Work out the finished part from the listing and answer in its coordinate system (mm). Round coordinates to 2 decimals unless told otherwise and drop trailing zeros. Order: outer loops, then holes, each group sorted by start corner. A loop starts at its lowest first (then second) coordinate and runs counter-clockwise, first axis right, second up. Notation, with made-up numbers: (48.5, -19.5) - (52.5, -19.5) arc R17 cw to (52.5, -1.5) - close; hole circle Ø4 at (88.5, 79). An arc over 180 degrees is marked (long way). Answer in a Markdown table with one row per item.
Autodesk Inventor part; units mm, degrees
ref_plane "YZ Plane" through (0, 0, 0) normal (1, 0, 0) x (0, 1, 0)
ref_plane "XZ Plane" through (0, 0, 0) normal (0, 1, 0) x (-1, 0, 0)
ref_plane "XY Plane" through (0, 0, 0) normal (0, 0, 1) x (1, 0, 0)
sketch "Sketch1" plane through (0, 0, 0) normal (0, 1, 0) x (-1, 0, 0)
  line L0 (0, 0) -> (40, 0)
  line L1 (40, 0) -> (40, -40)
  line L2 (40, -40) -> (0, -40)
  line L3 (0, -15.101) -> (0, 0)
  line L4 (0, -24.899) -> (0, -40)
  arc A0 (0, -24.899) -> (0, -15.101) centre (5.8365, -20) ccw
  dimension "d0" = 40
  dimension "d1" = 40
  dimension "d7" = 7.62
extrude "Extrusion1" add sketch "Sketch1" along normal blind 40
properties part number "railblock"
1) Find section C-C, the plane x = -3. Give the vertices of the cut face in (y, z).
Filled in:
| item | result |
|---|---|
| outline | (0, -40) - (40, -40) - (40, -27.07) - (0, -27.07) - close; (0, -12.93) - (40, -12.93) - (40, 0) - (0, 0) - close |
2) Find section A-A, the plane z = -27. Give the vertices of the cut face in (x, y), then the cut area to 3 significant figures.
Filled in:
| item | result |
|---|---|
| outline | (-40, 0) - (-8.85, 0) - (-8.85, 40) - (-40, 40) - close; (-2.83, 0) - (0, 0) - (0, 40) - (-2.83, 40) - close |
| area | 1,360 mm^2 |
3) Find section B-B, the plane y = 18.5. Give the vertices of the cut face in (x, z).
Filled in:
| item | result |
|---|---|
| outline | (-40, -40) - (0, -40) - (0, -24.9) arc R7.62 cw (long way) to (0, -15.1) - (0, 0) - (-40, 0) - close |
4) Find section D-D, the plane z = -20. Give the vertices of the cut face in (x, y).
Filled in:
| item | result |
|---|---|
| outline | (-40, 0) - (-13.46, 0) - (-13.46, 40) - (-40, 40) - close |
5) Find the intervals of material crossed by probe 1 along X at (y, z) = (31, -20); probe 2 along Z at (x, y) = (-3.5, 37); probe 3 along X at (y, z) = (13.5, -14.5), in increasing order. Write a range as from..to.
Filled in:
| item | result |
|---|---|
| probe 1 | x = -40..-13.46 |
| probe 2 | z = -40..-27.25, -12.75..0 |
| probe 3 | x = -40..-11.11, -0.56..0 |
6) The mould has two halves that part along Z. Classify faces 1 (the face through (-13.452, 19.72, -19.739)), 2 (the face through (0, 20, -8)), 3 (the face through (-20, 20, -40)), 4 (the face through (-20, 20, 0)): released by +Z, released by -Z, zero draft, split by the parting line, or undercut.
Filled in:
| item | result |
|---|---|
| face 1 | undercut |
| face 2 | zero draft |
| face 3 | released by -Z |
| face 4 | released by +Z |
